Design review of the part built by this model. Coordinates are the model's own, in mm. Round coordinates to 2 decimals unless told otherwise and drop trailing zeros. Loops run counter-clockwise (first coordinate to the right, second up) from the corner with the lowest first, then second, coordinate; pieces in that order, holes last. Notation, with made-up numbers: M 49.5,45.25 L 85.5,45.25 A9 cw 85.5,52.25 Z; hole C -9,77 d7. An arc over 180 degrees is marked long. Use a Markdown table: item, result.
from build123d import *

# Parameters (mm, degrees)
SKETCH1_R           = 3.302
BOSS_EXTRUDE1_DEPTH = 10.16


with BuildPart() as part:
    # Sketch1 → Boss-Extrude1 (new body)
    with BuildSketch(Plane(origin=(0, 0, 0), x_dir=(1, 0, 0), z_dir=(0, 1, 0))):
        Polygon((-25.4, 12.7), (25.4, 12.7), (25.4, 0), (76.2, 0), (76.2, -12.7), (25.4, -12.7), (-152.4, -12.7), (-152.4, 12.7), (-50.8, 12.7), (-50.8, 63.5), (-25.4, 63.5), align=None)
        with Locations(Location((0, 0, 0), (0, 0, 270))):
            Circle(SKETCH1_R, mode=Mode.SUBTRACT)
    extrude(amount=BOSS_EXTRUDE1_DEPTH)


solid = part.part
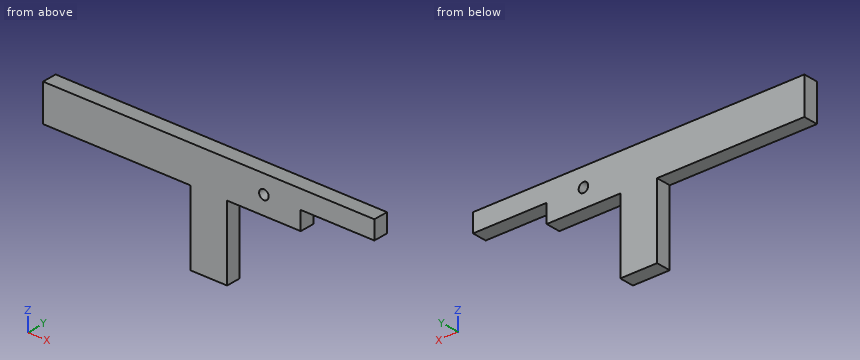
1. Take a section at B-B on y = 8.25. Give the boundary of the cut face in (x, z).
Check values:
| item | result |
|---|---|
| outline | M -152.4,-12.7 L -50.8,-12.7 L -50.8,-63.5 L -25.4,-63.5 L -25.4,-12.7 L 25.4,-12.7 L 25.4,0 L 76.2,0 L 76.2,12.7 L -152.4,12.7 Z; hole C 0,0 d6.6 |
2. Wall thickness on line 1 along X through (y, z) = (5.5, -46.5); line 2 along Z through (x, y) = (-115.5, 5.25); line 3 along Z through (x, y) = (54.5, 4.25): over which ranges is each line inside the solid? List them lowest first. Write a range as from..to.
Check values:
| item | result |
|---|---|
| line 1 | x = -50.8..-25.4 |
| line 2 | z = -12.7..12.7 |
| line 3 | z = 0..12.7 |
3. Take a section at C-C on z = -7.5. Give the boundary of the cut face in (x, y).
Check values:
| item | result |
|---|---|
| outline | M -152.4,0 L 25.4,0 L 25.4,10.16 L -152.4,10.16 Z |
4. Take a section at D-D on x = -128.5. Give the boundary of the cut face in (y, z).
Check values:
| item | result |
|---|---|
| outline | M 0,-12.7 L 10.16,-12.7 L 10.16,12.7 L 0,12.7 Z |
5. Insertion check: pin 1 (2 mm diameter, centred on x = 46, y = 5.5, fed in from -Z); pin 2 (6 mm diameter, centred on x = -70, y = 2, fed in from -Z); pin 3 (3 mm diameter, centred on y = 4, z = -3.5, fed in from +X). Each pin has a flat end and moves straight along its axis. Give the tip position at first contact, or say it passes through.
Check values:
| item | result |
|---|---|
| pin 1 | stops at z = 0 |
| pin 2 | stops at z = -12.7 |
| pin 3 | stops at x = 25.4 |
6. Take a section at A-A on x = 0. Give the boundary of the cut face in (y, z).
Check values:
| item | result |
|---|---|
| outline | M 0,-12.7 L 10.16,-12.7 L 10.16,-3.3 L 0,-3.3 Z; M 0,3.3 L 10.16,3.3 L 10.16,12.7 L 0,12.7 Z |
